Source: CAD feature listing. Evaluate the final solid. Frame: model axes, mm. Face numbers are marked on the shaded views. Give positions to 0.01 mm unless a question says otherwise; leave off trailing zeros. Loops run counter-clockwise (first coordinate to the right, second up) from the corner with the lowest first, then second, coordinate; pieces in that order, holes last.
```python
from build123d import *

# Parameters (mm, degrees)
SKETCH_1_R          = 60
SKETCH_1_R_2        = 20
EXTRUDE_1_DEPTH     = 5
SKETCH_4_W          = 210
SKETCH_4_H          = 125
SKETCH_4_R          = 60
EXTRUDE_2_DEPTH     = 5
SKETCH_5_R          = 2.2
CUT_EXTRUDE_2_DEPTH = 5
FILLET_1_R          = 15
SKETCH_2_R          = 2.75
CUT_EXTRUDE_3_DEPTH = 10


with BuildPart() as part:
    # 草图1 → 凸台-拉伸1 (new body)
    with BuildSketch(Plane(origin=(0, 0, 0), x_dir=(1, 0, 0), z_dir=(0, 1, 0))):
        with Locations(Location((0, 0, 0), (0, 0, 270))):
            Circle(SKETCH_1_R)
        with Locations(Location((0, 0, 0), (0, 0, 270))):
            Circle(SKETCH_1_R_2, mode=Mode.SUBTRACT)
    extrude(amount=EXTRUDE_1_DEPTH)

    # 草图4 → 凸台-拉伸2 (add)
    with BuildSketch(Plane(origin=(0, 0, 0), x_dir=(1, 0, 0), z_dir=(0, 1, 0))):
        Rectangle(SKETCH_4_W, SKETCH_4_H)
        Circle(SKETCH_4_R, mode=Mode.SUBTRACT)
    extrude(amount=EXTRUDE_2_DEPTH)

    # 草图5 → 切除-拉伸2 (cut)
    with BuildSketch(Plane(origin=(0, 5, 0), x_dir=(1, 0, 0), z_dir=(0, 1, 0))):
        with Locations(Location((-90, 47.5, 0), (0, 0, 270))):
            Circle(SKETCH_5_R)
        with Locations(Location((90, 47.5, 0), (0, 0, 90))):
            Circle(SKETCH_5_R)
        with Locations(Location((90, -47.5, 0), (0, 0, 270))):
            Circle(SKETCH_5_R)
        with Locations(Location((-90, -47.5, 0), (0, 0, 90))):
            Circle(SKETCH_5_R)
    extrude(amount=-CUT_EXTRUDE_2_DEPTH, mode=Mode.SUBTRACT)

    # 圆角1
    fillet_1_edges = [part.edges().sort_by_distance(p)[0] for p in [
        (-105, 2.5, -62.5),
        (-105, 2.5, 62.5),
        (105, 2.5, 62.5),
        (105, 2.5, -62.5),
    ]]
    fillet(fillet_1_edges, radius=FILLET_1_R)

    # 草图2 → 切除-拉伸3 (cut)
    with BuildSketch(Plane(origin=(0, 5, 0), x_dir=(1, 0, 0), z_dir=(0, 1, 0))):
        with Locations(Location((-23.57, 23.57, 0), (0, 0, 270))):
            Circle(SKETCH_2_R)
        with Locations(Location((23.57, 23.57, 0), (0, 0, 270))):
            Circle(SKETCH_2_R)
        with Locations(Location((23.57, -23.57, 0), (0, 0, 270))):
            Circle(SKETCH_2_R)
        with Locations(Location((-23.57, -23.57, 0), (0, 0, 270))):
            Circle(SKETCH_2_R)
    extrude(amount=-CUT_EXTRUDE_3_DEPTH, mode=Mode.SUBTRACT)


solid = part.part
```
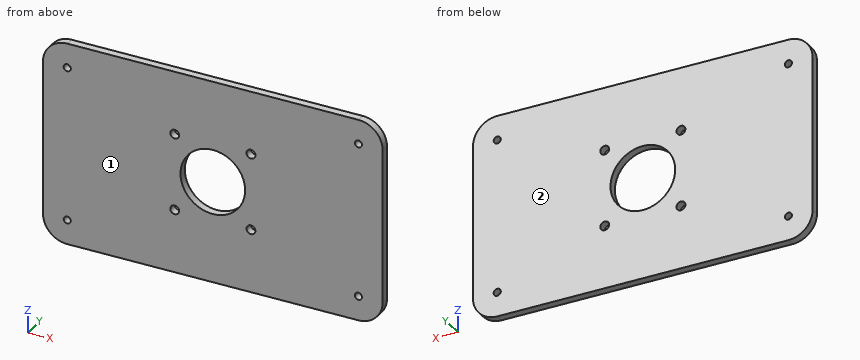
(1) Section B-B, the plane x = -23.57. Return the cut outline in (y, z), then the cut area to 3 significant figures.
A:
outline: (0, -62.5) - (5, -62.5) - (5, -26.32) - (0, -26.32) - close; (0, -20.82) - (5, -20.82) - (5, 20.82) - (0, 20.82) - close; (0, 26.32) - (5, 26.32) - (5, 62.5) - (0, 62.5) - close
area: 570 mm2
(2) First-contact query: pin 1 (5.5 mm diameter, centred on x = -90, z = 47.5, fed in from +Y); pin 2 (5 mm diameter, centred on x = 23.57, z = 23.57, fed in from +Y). Flat tips, straight axial feed; report the tip coordinate or a pass-through.
A:
pin 1: stops at y = 5
pin 2: passes through
(3) Ray query, line 1 along X through (y, z) = (3.6, -47.5); line 2 along X through (y, z) = (1.7, 23.57); line 3 along X through (y, z) = (1, 0). Return the intervals inside material, ascending.
A:
line 1: x = -105 to -92.2, -87.8 to 87.8, 92.2 to 105
line 2: x = -105 to -26.32, -20.82 to 20.82, 26.32 to 105
line 3: x = -105 to -20, 20 to 105
(4) Section C-C, the plane y = 2.3. Count the separate pieces of the cut face and the enclosed holes in it, then the cut area to 3 significant figures.
A:
separate pieces: 1
enclosed holes: 9
area: 24,600 mm2
(5) Section A-A, the plane z = 23.57. Return the cut outline in (x, y).
A:
outline: (-105, 0) - (-26.32, 0) - (-26.32, 5) - (-105, 5) - close; (-20.82, 0) - (20.82, 0) - (20.82, 5) - (-20.82, 5) - close; (26.32, 0) - (105, 0) - (105, 5) - (26.32, 5) - close
(6) Section D-D, the plane z = 0. Return the cut outline in (x, y), then the cut area to 3 significant figures.
A:
outline: (-105, 0) - (-20, 0) - (-20, 5) - (-105, 5) - close; (20, 0) - (105, 0) - (105, 5) - (20, 5) - close
area: 850 mm2
(7) Mould query, pull axis Y, two halves, no side actions, for the marked faces 1 and 2. Classes: pulls with the +Y half, pulls with the -Y half, needs draft (parallel to the pull), parting line crosses it, or undercut.
A:
face 1: pulls with the -Y half
face 2: pulls with the +Y half
